Check sheet for the drawn part. Datum: minimum x, y, z corner. Units: mm. A direction names the side the tool comes from. Coordinates: 2 decimals unless noted, no trailing zeros. Write each loop counter-clockwise with the first axis right and the second up, starting at its lowest first coordinate (ties: lowest second). Pieces come first, ordered by that corner, then holes. Notation, with made-up numbers: (-8.5, 26) - (4.5, 26) arc R33 ccw to (4.5, 57) - close; hole circle Ø2 at (51.25, -35). An arc over 180 degrees is marked (long way). Use CSV: the item, a comma, the result in double quotes. Start each with the question number.
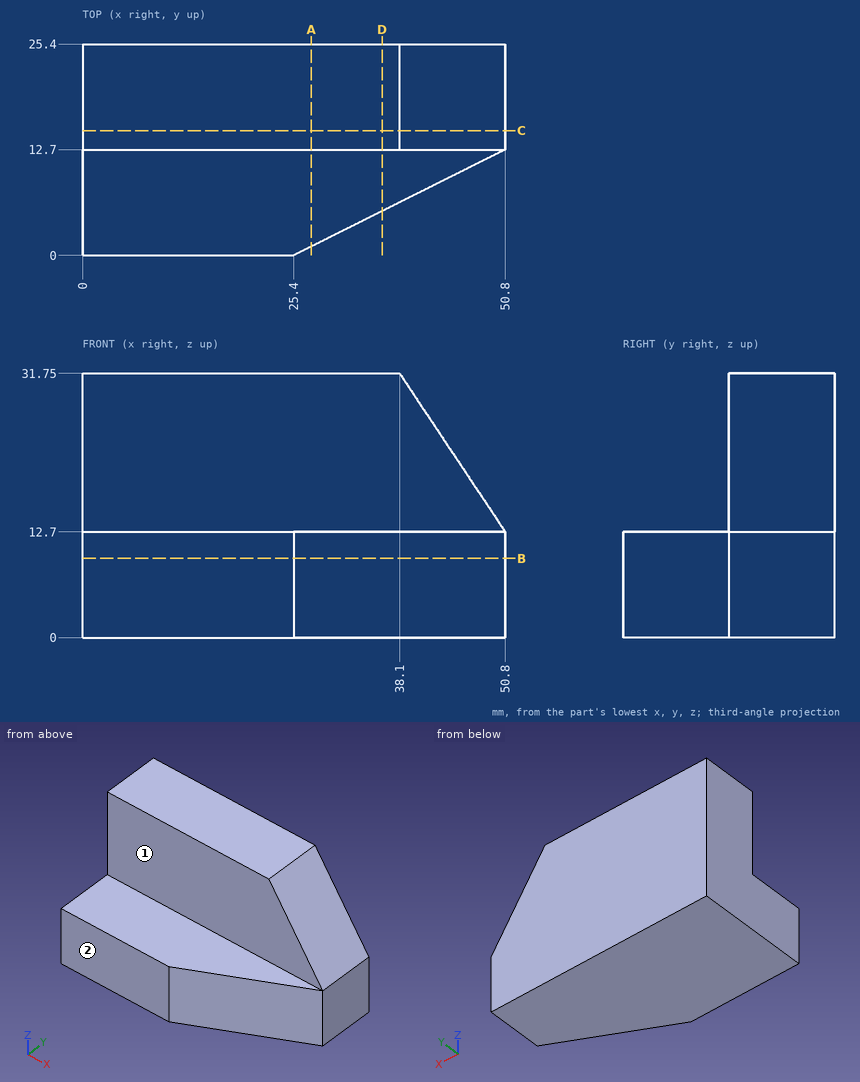
Q1. Cross-section at C-C (y = 15). Record the cut outline in (x, z).
Q2. Cross-section at D-D (x = 36). Record the cut outline in (y, z).
Q3. Tool access check on the marked faces 1 and 2. Record the directions out of +Z, -Z, +X, -X, +Y, -Y that give a thin tool (end or side, any length) a straight path to the whole face; none if there is none.
Q4. Cross-section at B-B (z = 9.5). Record the cut outline in (x, y), plus the area to 3 significant figures.
Q5. Cross-section at A-A (x = 27.5). Record the cut outline in (y, z), plus the area to 3 significant figures.
Q6. Gauge pin test, flat ends, axial feed: pin 1 (9.5 mm diameter, centred on x = 22.5, z = 26, fed in from -Y); pin 2 (3 mm diameter, centred on y = 12, z = 3.5, fed in from +X); pin 3 (4 mm diameter, centred on x = 31, y = 4.5, fed in from +Z); pin 4 (12 mm diameter, centred on y = 17.5, z = 22.5, fed in from +X). Record the tip position at first contact, or that the pin passes through.
Q7. Scan lines: line 1 along Y through (x, z) = (25, 13.5); line 2 along Z through (x, y) = (6, 7.25); line 3 along X through (y, z) = (8, 2). Record each from-to range of solid material in increasing order. Write a range as from..to.
Reply:
1,outline,"(0, 0) - (50.8, 0) - (50.8, 12.7) - (38.1, 31.75) - (0, 31.75) - close"
2,outline,"(5.3, 0) - (25.4, 0) - (25.4, 31.75) - (12.7, 31.75) - (12.7, 12.7) - (5.3, 12.7) - close"
3,face 1,"+Z, +X, -X, -Y"
3,face 2,"+Z, -Z, +X, -X, -Y"
4,outline,"(0, 0) - (25.4, 0) - (50.8, 12.7) - (50.8, 25.4) - (0, 25.4) - close"
4,area,"1,130 mm^2"
5,outline,"(1.05, 0) - (25.4, 0) - (25.4, 31.75) - (12.7, 31.75) - (12.7, 12.7) - (1.05, 12.7) - close"
5,area,"551 mm^2"
6,pin 1,"y = 12.7"
6,pin 2,"x = 50.8"
6,pin 3,"z = 12.7"
6,pin 4,"x = 48.27"
7,line 1,"12.7..25.4"
7,line 2,"0..12.7"
7,line 3,"0..41.4"
